from build123d import *

# Parameters (mm, degrees)
SKETCH2_W               = 25
SKETCH2_H               = 9
BOSS_EXTRUDE3_DEPTH     = 6
SKETCH3_R               = 2.55
CUT_EXTRUDE1_DEPTH      = 5
CUT_EXTRUDE2_DEPTH      = 28.239676944
CUT_EXTRUDE2_DEPTH_BACK = 28.239676944
SKETCH4_R               = 1.5
SKETCH5_R               = 1.5
CUT_EXTRUDE3_DEPTH      = 4.5
CUT_EXTRUDE4_DEPTH      = 28.239676944
FILLET2_R               = 0.4
SKETCH8_R               = 1
CUT_EXTRUDE5_DEPTH      = 28.239676944
CUT_EXTRUDE7_DEPTH      = 10


with BuildPart() as part:
    # Sketch2 → Boss-Extrude3 (new body)
    with BuildSketch(Plane(origin=(0, 0, 0), x_dir=(1, 0, 0), z_dir=(0, 1, 0))):
        with Locations((12.5, 4.5)):
            Rectangle(SKETCH2_W, SKETCH2_H)
    extrude(amount=BOSS_EXTRUDE3_DEPTH)

    # Sketch3 → Cut-Extrude1 (cut)
    with BuildSketch(Plane(origin=(0, 6, 0), x_dir=(1, 0, 0), z_dir=(0, 1, 0))):
        with Locations(Location((4.5, 4.5, 0), (0, 0, 270))):
            Circle(SKETCH3_R)
    extrude(amount=-CUT_EXTRUDE1_DEPTH, mode=Mode.SUBTRACT)

    # Sketch4 → Cut-Extrude2 (cut, two sides: drawn at the far end of the back side and taken through both)
    with BuildSketch(Plane(origin=(0, 6, 0), x_dir=(1, 0, 0), z_dir=(0, 1, 0)).offset(-CUT_EXTRUDE2_DEPTH_BACK)):
        with Locations(Location((22.25, 4.5, 0), (0, 0, 270))):
            Circle(SKETCH4_R)
    extrude(amount=CUT_EXTRUDE2_DEPTH + CUT_EXTRUDE2_DEPTH_BACK, mode=Mode.SUBTRACT)

    # Sketch5 → Cut-Extrude3 (cut)
    with BuildSketch(Plane(origin=(0, 6, 0), x_dir=(1, 0, 0), z_dir=(0, 1, 0))):
        with BuildLine():
            Line((25, 9), (4.5, 9))
            ThreePointArc((4.5, 9), (7.681980515, 7.681980515), (9, 4.5))
            ThreePointArc((9, 4.5), (7.681980515, 1.318019485), (4.5, 0))
            Line((4.5, 0), (25, 0))
            Line((25, 0), (25, 9))
        make_face()
        with Locations(Location((22.25, 4.5, 0), (0, 0, 270))):
            Circle(SKETCH5_R, mode=Mode.SUBTRACT)
    extrude(amount=-CUT_EXTRUDE3_DEPTH, mode=Mode.SUBTRACT)

    # Sketch6 → Cut-Extrude4 (cut, through all)
    with BuildSketch(Plane(origin=(0, 6, 0), x_dir=(1, 0, 0), z_dir=(0, 1, 0))):
        with BuildLine():
            ThreePointArc((0, 4.5), (1.318019485, 7.681980515), (4.5, 9))
            Line((4.5, 9), (0, 9))
            Line((0, 9), (0, 4.5))
        make_face()
        with BuildLine():
            ThreePointArc((4.5, 0), (1.318019485, 1.318019485), (0, 4.5))
            Line((0, 4.5), (0, 0))
            Line((0, 0), (4.5, 0))
        make_face()
    extrude(amount=-CUT_EXTRUDE4_DEPTH, mode=Mode.SUBTRACT)

    # Fillet2
    fillet2_edges = [part.edges().sort_by_distance(p)[0] for p in [
        (4.5, 6, -7.05),
    ]]
    fillet(fillet2_edges, radius=FILLET2_R)

    # Sketch8 → Cut-Extrude5 (cut, through all)
    with BuildSketch(Plane.XZ):
        with Locations(Location((4.5, -4.5, 0), (0, 0, 270))):
            Circle(SKETCH8_R)
    extrude(amount=-CUT_EXTRUDE5_DEPTH, mode=Mode.SUBTRACT)

    # Sketch9 → Cut-Extrude7 (cut)
    with BuildSketch(Plane(origin=(0, 1.5, 0), x_dir=(1, 0, 0), z_dir=(0, 1, 0))):
        with BuildLine():
            Line((25, 9), (4.5, 9))
            ThreePointArc((4.5, 9), (6.291176984, 8.628157581), (7.786338153, 7.574082228))
            ThreePointArc((7.786338153, 7.574082228), (14.648850695, 6.181991531), (21.61241808, 6.917331027))
            ThreePointArc((21.61241808, 6.917331027), (24.75, 4.499999954), (21.612417992, 2.082668996))
            ThreePointArc((21.612417992, 2.082668996), (14.64885065, 2.818008467), (7.786338153, 1.425917772))
            ThreePointArc((7.786338153, 1.425917772), (6.291176984, 0.371842419), (4.5, 0))
            Line((4.5, 0), (25, 0))
            Line((25, 0), (25, 9))
        make_face()
    extrude(amount=-CUT_EXTRUDE7_DEPTH, mode=Mode.SUBTRACT)


solid = part.part
The listing builds one solid part. Answer for the finished solid, in the listing's coordinates (mm). A direction names the side the tool comes from. Coordinates: 2 decimals unless noted, no trailing zeros. Write each loop counter-clockwise with the first axis right and the second up, starting at its lowest first coordinate (ties: lowest second). Pieces come first, ordered by that corner, then holes. Notation, with made-up numbers: M 17,32 L 71,32 A31 ccw 71,58 Z; hole C 17,45 d9. An arc over 180 degrees is marked long. Put each result on its own line as item: value. Start each with the question number.
1. A cutting plane is placed at C-C on y = 0.65. Write down the section's boundary in (x, z), then the cut area to 3 significant figures.
2. Flat-ended cylindrical pins translate along their axes: P1, Ø2.5, axis at x = 4.5, z = -3.5, coming from the +Y side; P2, Ø1, axis at x = 16, y = 1.5, coming from the +Z side; P3, Ø3, axis at x = 13, z = -3.5, coming from the +Y side. Find the tip coordinate at first contact, or state that the pin passes through.
3. Consider line 1 (X direction, y = 2.75, z = -4.5); line 2 (Y direction, x = 11, z = -3.5); line 3 (Z direction, x = 7.5, y = 2.8). Determine where each line is inside the solid, lowest interval first. Write a range as from..to.
4. A cutting plane is placed at A-A on x = 22.25. Write down the section's boundary in (y, z).
5. Which of the six approach directions +Z, -Z, +X, -X, +Y, -Y give full straight-line access (tool end or side, diameter ignored) to faces 4 (the cylindrical face through (23.737, 0.739, -4.695)), 5 (the cylindrical face through (5, 3, -2))?
6. For a pull along X with two mould halves and no side action, classify faces 1 (the cylindrical face through (14.551, 0.76, -6.187)), 2 (the flat face through (9, 0, -5)), 3 (the flat face through (5, 1, -3)) as pulls with the +X half, pulls with the -X half, needs draft (parallel to the pull), parting line crosses it, or undercut.
7. A cutting plane is placed at D-D on z = -5. Count the separate pieces of the cut face and the enclosed holes in it, then the cut area to 3 significant figures.
8. A cutting plane is placed at B-B on y = 3.5. Write down the section's boundary in (x, z).
Resolved:
1. outline: M 7.79,-7.57 A23.02 cw 21.61,-6.92 A2.5 ccw long 21.61,-2.08 A23.02 cw 7.79,-1.43 A4.5 ccw long Z; hole C 4.5,-4.5 d2; hole C 22.25,-4.5 d3
1. area: 117 mm2
2. P1: stops at y = 1
2. P2: stops at z = -2.83
2. P3: stops at y = 1.5
3. line 1: x = 0..1.95, 7.05..9
3. line 2: y = 0..1.5
3. line 3: z = -7.85..-1.15
4. outline: M 0,-7 L 1.5,-7 L 1.5,-6 L 0,-6 Z; M 0,-3 L 1.5,-3 L 1.5,-2 L 0,-2 Z
5. face 4: +Y, -Y
5. face 5: +Y
6. face 1: undercut
6. face 2: needs draft
6. face 3: undercut
7. separate pieces: 3
7. enclosed holes: 0
7. area: 46.2 mm2
8. outline: C 4.5,-4.5 d9; hole C 4.5,-4.5 d5.1
